Geometry: see drawing. Coordinates: mm, zero at the bounding-box minimum. Coordinates: 2 decimals unless noted, no trailing zeros. Order: outer loops, then holes, each group sorted by start corner. A loop starts at its lowest first (then second) coordinate and runs counter-clockwise, first axis right, second up.
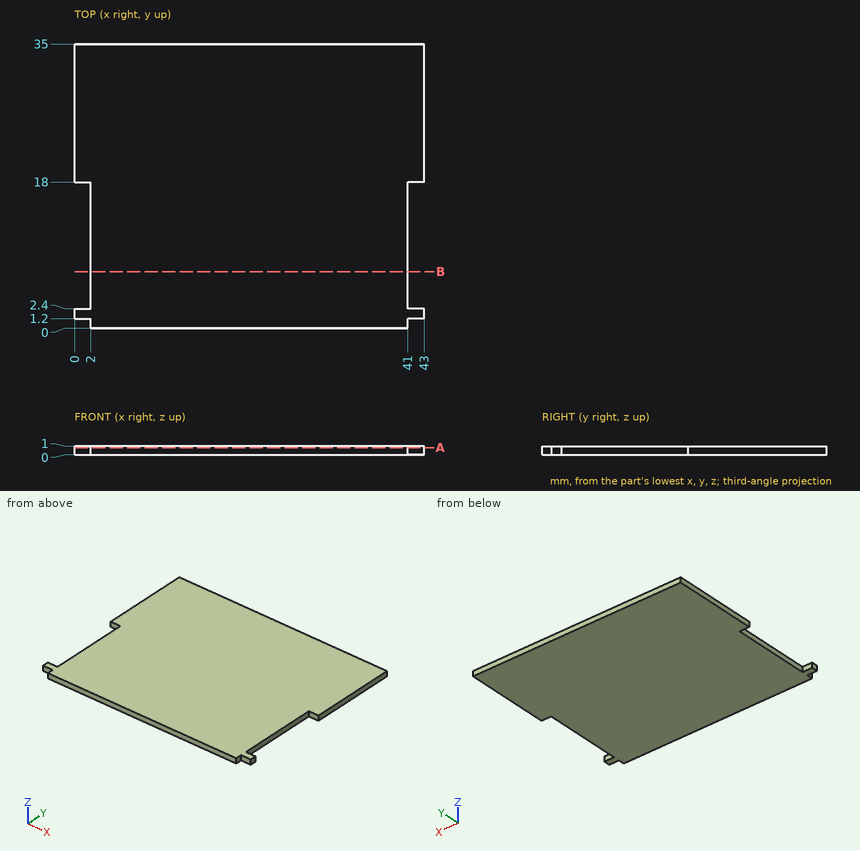
Item 1: Cut plane B-B on y = 7. Return loops of the section in (x, z).
Response values:
outline: (2, 0) - (41, 0) - (41, 1) - (2, 1) - close
Item 2: Cut plane A-A on z = 0.85. Return loops of the section in (x, y).
Response values:
outline: (0, 1.2) - (2, 1.2) - (2, 0) - (41, 0) - (41, 1.2) - (43, 1.2) - (43, 2.4) - (41, 2.4) - (41, 18) - (43, 18) - (43, 35) - (0, 35) - (0, 18) - (2, 18) - (2, 2.4) - (0, 2.4) - close
Item 3: Pin query (flat end, axial travel): pin 1 Ø8 at (x, y) = (28, 24.5) entering from -Z; pin 2 Ø0.5 at (y, z) = (8, 0.5) entering from -X; pin 3 Ø0.5 at (x, z) = (1, 0.5) entering from -Y. Return the tip coordinate at first contact, or that it passes through.
Response values:
pin 1: stops at z = 0
pin 2: stops at x = 2
pin 3: stops at y = 1.2
Item 4: Ray query, probe 1 along X at (y, z) = (10, 0.3). Return the intervals inside material, ascending.
Response values:
probe 1: x = 2 to 41
